Can you work these out from the model? Positions are in its coordinate system, mm. Face numbers are marked on the shaded views. A direction names the side the tool comes from. Round coordinates to 2 decimals unless told otherwise and drop trailing zeros. Order: outer loops, then holes, each group sorted by start corner. A loop starts at its lowest first (then second) coordinate and runs counter-clockwise, first axis right, second up.
Q1. For the marked faces 1, 2 and 3, which set-ups out of +Z, -Z, +X, -X, +Y, -Y let a thin tool reach every point of the face, with its end or its side?
Q2. We'd pull the mould along X, two halves only. Please class the marked faces 4, 5, 6 and 7: pulls with the +X half, pulls with the -X half, needs draft (parallel to the pull), parting line crosses it, or undercut.
Q3. If we section it at A-A (z = 35): Please give me the cut outline in (x, y) (1 decimal), plus the area to 3 significant figures.
Q4. Will these pins go through, and if not, where does the flat tip stop? P1, Ø18.5, axis at x = -38.5, y = 4, coming from the +Z side; P2, Ø3.5, axis at y = 0, z = 33.5, coming from the +X side; P3, Ø1, axis at x = -38, y = 17, coming from the +Z side.
Q5. If I drill on line 1 (X direction, y = -2.5, z = 38); line 2 (X direction, y = -28, z = 35); line 3 (Z direction, x = 48, y = -23), over which ranges is the centre line in solid material (lowest first)?
Q6. If we section it at B-B (x = -43): Please give me the cut outline in (y, z) (3 decimals).
Q7. If we section it at C-C (z = 52.5): Please give me the cut outline in (x, y) (1 decimal), plus the area to 3 significant figures.
Q8. If we section it at D-D (x = -22): Please give me the cut outline in (y, z) (3 decimals), plus the area to 3 significant figures.
from build123d import *

# Parameters (mm, degrees)
SKETCH1_W                   = 119.7483
SKETCH1_H                   = 67.31
BOSS_EXTRUDE1_DEPTH         = 26.2382
SKETCH2_R                   = 31.0515
BOSS_EXTRUDE2_DEPTH         = 30.48
CHAMFER1_SIZE               = 2.54
SKETCH3_W                   = 35.56
SKETCH3_H                   = 67.31
BOSS_EXTRUDE3_DEPTH         = 18.288
CHAMFER2_SIZE               = 17.78
CHAMFER2_SIZE2              = 9.144
FILLET1_R                   = 6.35
CUT_EXTRUDE1_DEPTH          = 0.254
F_1_4_20_TAPPED_HOLE1_D     = 5.1054
F_1_4_20_TAPPED_HOLE1_DEPTH = 16.51
F_1_4_20_TAPPED_HOLE1_TIP   = 1.533816902


with BuildPart() as part:
    # Sketch1 → Boss-Extrude1 (new body)
    with BuildSketch(Plane.XY):
        Rectangle(SKETCH1_W, SKETCH1_H)
    extrude(amount=BOSS_EXTRUDE1_DEPTH)

    # Sketch2 → Boss-Extrude2 (add)
    with BuildSketch(Plane.XY.offset(26.2382)):
        with Locations(Location((18.66265, -2.6035, 0), (0, 0, 270))):
            Circle(SKETCH2_R)
    extrude(amount=BOSS_EXTRUDE2_DEPTH)

    # Chamfer1
    chamfer1_edges = [part.edges().sort_by_distance(p)[0] for p in [
        (18.66265, 28.448, 56.7182),
    ]]
    chamfer(chamfer1_edges, length=CHAMFER1_SIZE)

    # Sketch3 → Boss-Extrude3 (add)
    with BuildSketch(Plane.XY.offset(26.2382)):
        with Locations((-42.09415, 0)):
            Rectangle(SKETCH3_W, SKETCH3_H)
    extrude(amount=BOSS_EXTRUDE3_DEPTH)

    # Chamfer2
    chamfer2_edges = [part.edges().sort_by_distance(p)[0] for p in [
        (-42.09415, 33.655, 44.5262),
    ]]
    chamfer2_side = [part.faces().sort_by_distance(p)[0] for p in [
        (-7.218498902, 33.655, 16.936879024),
    ]]
    chamfer(chamfer2_edges, length=CHAMFER2_SIZE, length2=CHAMFER2_SIZE2, reference=chamfer2_side[0])

    # Fillet1
    fillet1_edges = [part.edges().sort_by_distance(p)[0] for p in [
        (-24.31415, -4.572, 44.5262),
        (-59.87415, -4.572, 44.5262),
        (-42.09415, 24.511, 44.5262),
    ]]
    fillet(fillet1_edges, radius=FILLET1_R)

    # Sketch4 → Cut-Extrude1 (cut)
    with BuildSketch(Plane.XY.offset(44.5262)):
        with BuildLine():
            Line((-39.36365, 18.892871189), (-34.063036375, 18.892871189))
            ThreePointArc((-34.063036375, 18.892871189), (-32.427100781, 17.256935594), (-34.063036375, 15.621))
            Line((-34.063036375, 15.621), (-39.36365, 15.621))
            ThreePointArc((-39.36365, 15.621), (-40.999585594, 17.256935594), (-39.36365, 18.892871189))
        make_face()
    extrude(amount=-CUT_EXTRUDE1_DEPTH, mode=Mode.SUBTRACT)

    # 1/4-20 Tapped Hole1
    with Locations(Plane(origin=(0, -33.655, 0), x_dir=(-1, 0, 0), z_dir=(0, -1, 0))):
        with Locations((-19.74215, -13.462)):
            Hole(F_1_4_20_TAPPED_HOLE1_D / 2, depth=F_1_4_20_TAPPED_HOLE1_DEPTH)
            with Locations((0, 0, -(F_1_4_20_TAPPED_HOLE1_DEPTH + F_1_4_20_TAPPED_HOLE1_TIP / 2))):  # 118° drill point
                Cone(0, F_1_4_20_TAPPED_HOLE1_D / 2, F_1_4_20_TAPPED_HOLE1_TIP, mode=Mode.SUBTRACT)


solid = part.part
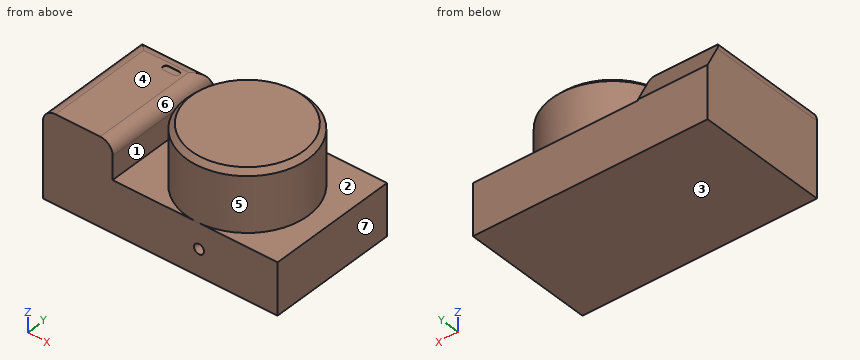
Solution:
1. face 1: +Z, +Y, -Y
1. face 2: +Z
1. face 3: -Z, +X, -X, +Y, -Y
2. face 4: needs draft
2. face 5: undercut
2. face 6: undercut
2. face 7: pulls with the +X half
3. outline: (-59.9, -33.7) - (-24.3, -33.7) - (-24.3, 29.4) - (-59.9, 29.4) - close; circle Ø62.1 at (18.7, -2.6)
3. area: 5,270 mm2
4. P1: stops at z = 44.53
4. P2: stops at x = 49.7
4. P3: stops at z = 44.27
5. line 1: x = -59.87 to -24.31, -12.39 to 49.71
5. line 2: x = -59.87 to -24.31, 0.8 to 36.53
5. line 3: z = 0 to 26.24
6. outline: (-33.655, 0) - (33.655, 0) - (33.655, 26.746) - (26.283, 41.08) arc R6.35 ccw to (20.636, 44.526) - (-33.655, 44.526) - close
7. outline: circle Ø62.1 at (18.7, -2.6)
7. area: 3,030 mm2
8. outline: (-33.655, 0) - (33.655, 0) - (33.655, 26.238) - (-33.655, 26.238) - close
8. area: 1,770 mm2
